Here's how the part is built. I have some questions about the finished solid (model axes, mm). A direction names the side the tool comes from. Round coordinates to 2 decimals unless told otherwise and drop trailing zeros. Loops run counter-clockwise (first coordinate to the right, second up) from the corner with the lowest first, then second, coordinate; pieces in that order, holes last. Notation, with made-up numbers: M -9,89 L 5,89 A32 cw 5,125 Z; hole C -23.5,-14 d6. An arc over 180 degrees is marked long. Answer as a JSON object with one key per item and string values.
from build123d import *

# Parameters (mm, degrees)
ESQUISSE1_W                     = 30
ESQUISSE1_H                     = 55
PLAQUE_PLEXI_DEPTH              = 6
PASSAGE_JAUGE_LAITON_REACH      = 33.894
ESQUISSE5_R                     = 7.5
PASSAGE_CROU_M5_REACH           = 33.894
ESQUISSE6_R                     = 2.65
ESQUISSE2_R                     = 12.2
ESQUISSE2_R_2                   = 9.8
GORGE_JOINT_CENTRAL_DEPTH       = 1.2
ESQUISSE7_R                     = 5.25
ESQUISSE7_R_2                   = 3.75
ENL_V_DE_MAT_EXTRU_MINCE2_DEPTH = 0.75
CONG_1_R                        = 3


with BuildPart() as part:
    # Esquisse1 → Plaque Plexi (new body)
    with BuildSketch(Plane(origin=(0, 0, 0), x_dir=(1, 0, 0), z_dir=(0, 1, 0))):
        Rectangle(ESQUISSE1_W, ESQUISSE1_H)
    extrude(amount=PLAQUE_PLEXI_DEPTH)

    # Esquisse5 → Passage Jauge Laiton (cut, up to next)
    with BuildSketch(Plane(origin=(0, 6, 0), x_dir=(1, 0, 0), z_dir=(0, 1, 0)), mode=Mode.PRIVATE) as passage_jauge_laiton_sk1:
        with Locations(Location((0, 0, 0), (0, 0, 270))):
            Circle(ESQUISSE5_R)
    passage_jauge_laiton_tool1 = extrude(passage_jauge_laiton_sk1.sketch, amount=-PASSAGE_JAUGE_LAITON_REACH, mode=Mode.PRIVATE) & part.part
    add(passage_jauge_laiton_tool1.solids().sort_by_distance((0, 6, 0))[0], mode=Mode.SUBTRACT)

    # Esquisse6 → Passage écrou M5 (cut, up to next)
    with BuildSketch(Plane(origin=(0, 6, 0), x_dir=(1, 0, 0), z_dir=(0, 1, 0)), mode=Mode.PRIVATE) as passage_crou_m5_sk1:
        with Locations(Location((0, 20, 0), (0, 0, 270))):
            Circle(ESQUISSE6_R)
    passage_crou_m5_tool1 = extrude(passage_crou_m5_sk1.sketch, amount=-PASSAGE_CROU_M5_REACH, mode=Mode.PRIVATE) & part.part
    # Esquisse6 → Passage écrou M5 (cut, up to next)
    with BuildSketch(Plane(origin=(0, 6, 0), x_dir=(1, 0, 0), z_dir=(0, 1, 0)), mode=Mode.PRIVATE) as passage_crou_m5_sk2:
        with Locations(Location((0, -20, 0), (0, 0, 270))):
            Circle(ESQUISSE6_R)
    passage_crou_m5_tool2 = extrude(passage_crou_m5_sk2.sketch, amount=-PASSAGE_CROU_M5_REACH, mode=Mode.PRIVATE) & part.part
    add(passage_crou_m5_tool1.solids().sort_by_distance((0, 6, -20))[0], mode=Mode.SUBTRACT)
    add(passage_crou_m5_tool2.solids().sort_by_distance((0, 6, 20))[0], mode=Mode.SUBTRACT)

    # Esquisse2 → Gorge_Joint_central (cut)
    with BuildSketch(Plane(origin=(0, 6, 0), x_dir=(1, 0, 0), z_dir=(0, 1, 0))):
        Circle(ESQUISSE2_R)
        Circle(ESQUISSE2_R_2, mode=Mode.SUBTRACT)
    extrude(amount=-GORGE_JOINT_CENTRAL_DEPTH, mode=Mode.SUBTRACT)

    # Esquisse7 → Enlèv. de mat.-Extru.-Mince2 (cut)
    # profile 1 of 2: a face of its own
    with BuildSketch(Plane(origin=(0, 6, 0), x_dir=(1, 0, 0), z_dir=(0, 1, 0))):
        with Locations((0, -20)):
            Circle(ESQUISSE7_R)
        with Locations((0, -20)):
            Circle(ESQUISSE7_R_2, mode=Mode.SUBTRACT)
    # profile 2 of 2: a face of its own
    with BuildSketch(Plane(origin=(0, 6, 0), x_dir=(1, 0, 0), z_dir=(0, 1, 0))):
        with Locations((0, 20)):
            Circle(ESQUISSE7_R)
        with Locations((0, 20)):
            Circle(ESQUISSE7_R_2, mode=Mode.SUBTRACT)
    extrude(amount=-ENL_V_DE_MAT_EXTRU_MINCE2_DEPTH, mode=Mode.SUBTRACT)

    # Congé1
    cong_1_edges = [part.edges().sort_by_distance(p)[0] for p in [
        (-15, 3, -27.5),
        (15, 3, -27.5),
        (15, 3, 27.5),
        (-15, 3, 27.5),
    ]]
    fillet(cong_1_edges, radius=CONG_1_R)


solid = part.part
Item 1: I want a section at C-C, the plane x = 0. State how many separate pieces and enclosed holes the cut face has, then the cut area to 3 significant figures.
Resolved:
{"separate pieces": "4", "enclosed holes": "0", "area": "166 mm²"}
Item 2: I want a section at A-A, the plane z = 0. Please give me the cut outline in (x, y).
Resolved:
{"outline": "M -15,0 L -7.5,0 L -7.5,6 L -9.8,6 L -9.8,4.8 L -12.2,4.8 L -12.2,6 L -15,6 Z; M 7.5,0 L 15,0 L 15,6 L 12.2,6 L 12.2,4.8 L 9.8,4.8 L 9.8,6 L 7.5,6 Z"}
Item 3: Please list where these lines run through material, in increasing order: probe 1 along Z at (x, y) = (0.25, 2.05); probe 2 along X at (y, z) = (5.5, 0); probe 3 along X at (y, z) = (1.55, 0). Write a range as from..to.
Resolved:
{"probe 1": "-27.5..-22.64, -17.36..-7.5, 7.5..17.36, 22.64..27.5", "probe 2": "-15..-12.2, -9.8..-7.5, 7.5..9.8, 12.2..15", "probe 3": "-15..-7.5, 7.5..15"}
Item 4: I want a section at D-D, the plane z = 20. Please give me the cut outline in (x, y).
Resolved:
{"outline": "M -15,0 L -2.65,0 L -2.65,6 L -3.75,6 L -3.75,5.25 L -5.25,5.25 L -5.25,6 L -15,6 Z; M 2.65,0 L 15,0 L 15,6 L 5.25,6 L 5.25,5.25 L 3.75,5.25 L 3.75,6 L 2.65,6 Z"}
Item 5: On a 3-axis mill with a long thin cutter (end or side, diameter ignored), from which of +Z, -Z, +X, -X, +Y, -Y can I reach the whole of each face in a straight line? I mean faces 4 (the face through (-7, 0, -6)), 5 (the face through (-0.81, 5.63, 23.66)). Say none if no direction works.
Resolved:
{"face 4": "+Z, -Z, +X, -X, -Y", "face 5": "+Y"}
Item 6: If we mould it in two halves opening along X, with no side actions, what happens to faces 1 (the face through (-12.19, 5.41, -0.54)), 2 (the face through (14.1, 3.04, 26.64)), 3 (the face through (-14.14, 3.04, 26.6))? For each: pulls with the +X half, pulls with the -X half, needs draft (parallel to the pull), parting line crosses it, or undercut.
Resolved:
{"face 1": "undercut", "face 2": "pulls with the +X half", "face 3": "pulls with the -X half"}
Item 7: I want a section at B-B, the plane y = 2.35. Please give me the cut outline in (x, z).
Resolved:
{"outline": "M -15,-24.5 A3 ccw -12,-27.5 L 12,-27.5 A3 ccw 15,-24.5 L 15,24.5 A3 ccw 12,27.5 L -12,27.5 A3 ccw -15,24.5 Z; hole C 0,0 d15; hole C 0,-20 d5.3; hole C 0,20 d5.3"}
